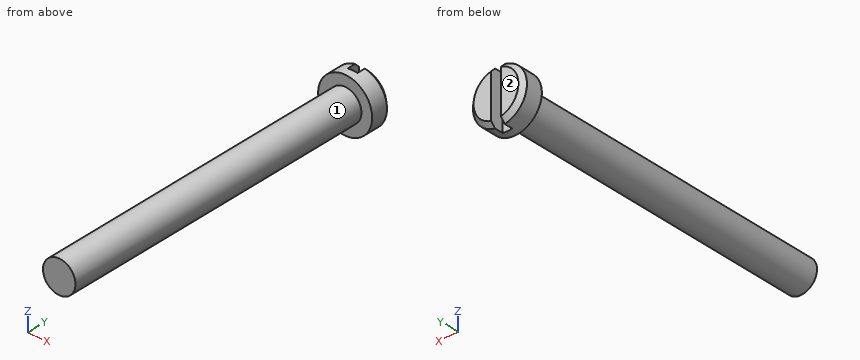
```python
from build123d import *

# Parameters (mm, degrees)
CHAMFER1_SIZE           = 0.7
SKETCH2_W               = 1.5
SKETCH2_H               = 6.7872108
CUT_EXTRUDE1_DEPTH      = 50
CUT_EXTRUDE1_DEPTH_BACK = 19


with BuildPart() as part:
    # Sketch1 → Revolve1 (revolve)
    with BuildSketch(Plane.XY):
        Polygon((0, 53.3), (4.15, 53.3), (4.15, 50), (2.5, 50), (2.5, 0), (0, 0), (0, 50), align=None)
    revolve(axis=Axis((0, 0, 0), (0, 1, 0)))

    # Chamfer1
    chamfer1_edges = [part.edges().sort_by_distance(p)[0] for p in [
        (-4.15, 53.3, 0),
    ]]
    chamfer(chamfer1_edges, length=CHAMFER1_SIZE)

    # Sketch2 → Cut-Extrude1 (cut, two sides)
    with BuildSketch(Plane.XY) as cut_extrude1_sk:
        with Locations((0.003512463, 54.6936054)):
            Rectangle(SKETCH2_W, SKETCH2_H)
    extrude(amount=CUT_EXTRUDE1_DEPTH, mode=Mode.SUBTRACT)
    extrude(cut_extrude1_sk.sketch, amount=-CUT_EXTRUDE1_DEPTH_BACK, mode=Mode.SUBTRACT)


solid = part.part
```
Part model, mm, in its own coordinate system. Face numbers are marked on the shaded views. A direction names the side the tool comes from. Round coordinates to 2 decimals unless told otherwise and drop trailing zeros. Write each loop counter-clockwise with the first axis right and the second up, starting at its lowest first coordinate (ties: lowest second). Pieces come first, ordered by that corner, then holes. Notation, with made-up numbers: M 29.5,45 L 51.5,45 A13 cw 51.5,56 Z; hole C 80.5,-28 d2. An arc over 180 degrees is marked long. One line per question, with ' | ' between items.
(1) Probe line 1 along Y through (x, z) = (-1.5, 2.75); line 2 along Y through (x, z) = (-0.25, -1.5); line 3 along X through (y, z) = (6, 2.25). List the from-to ranges inside material, lowest first.
Answer key:
line 1: y = 50 to 53.3 | line 2: y = 0 to 51.3 | line 3: x = -1.09 to 1.09
(2) Saw through at B-B on y = 6. Write the cut outline in (x, z), then the cut area to 3 significant figures.
Answer key:
outline: C 0,0 d5 | area: 19.6 mm^2
(3) Pin check, flat tips, straight feed: pin 1 (0.6 mm diameter, centred on y = 52, z = 0.5, fed in from -X); pin 2 (0.5 mm diameter, centred on x = 0, z = -1.5, fed in from +Y); pin 3 (4 mm diameter, centred on x = 0, y = 12.5, fed in from -Z). Stop position of each tip, or through.
Answer key:
pin 1: stops at x = -4.15 | pin 2: stops at y = 51.3 | pin 3: stops at z = -2.5
(4) Saw through at A-A on z = 0. Write the cut outline in (x, y).
Answer key:
outline: M -4.15,50 L -2.5,50 L -2.5,0 L 2.5,0 L 2.5,50 L 4.15,50 L 4.15,52.6 L 3.45,53.3 L 0.75,53.3 L 0.75,51.3 L -0.75,51.3 L -0.75,53.3 L -3.45,53.3 L -4.15,52.6 Z
(5) 3-axis set-ups, long thin cutter, end or side, ignore diameter. For the marked faces 1 and 2: which of +Z, -Z, +X, -X, +Y, -Y reach the whole face in a straight line?
Answer key:
face 1: -Y | face 2: +Z, -Z, +X, -X, +Y
